from build123d import *

# Parameters (mm, degrees)
SKETCH1_R           = 10
BOSS_EXTRUDE1_DEPTH = 10


with BuildPart() as part:
    # Sketch1 → Boss-Extrude1 (new, symmetric)
    with BuildSketch(Plane.XY):
        with BuildLine():
            Line((-24.140215409, 6.5), (-11.587303396, 53.12))
            ThreePointArc((-11.587303396, 53.12), (0, 62), (11.587303396, 53.12))
            Line((11.587303396, 53.12), (24.140215409, 6.5))
            ThreePointArc((24.140215409, 6.5), (24.936514863, 1.780512988), (24.81883517, -3.004233816))
            ThreePointArc((24.81883517, -3.004233816), (30.762049538, -19.776348187), (47.717387131, -25.174694658))
            ThreePointArc((47.717387131, -25.174694658), (61.713032142, -49.370425713), (35.03522611, -41.027395935))
            ThreePointArc((35.03522611, -41.027395935), (26.046643252, -25.670606045), (8.378996809, -23.554031767))
            ThreePointArc((8.378996809, -23.554031767), (0, -25), (-8.378996809, -23.554031767))
            ThreePointArc((-8.378996809, -23.554031767), (-26.046643252, -25.670606045), (-35.03522611, -41.027395935))
            ThreePointArc((-35.03522611, -41.027395935), (-61.713032142, -49.370425713), (-47.717387131, -25.174694658))
            ThreePointArc((-47.717387131, -25.174694658), (-30.762049538, -19.776348187), (-24.81883517, -3.004233816))
            ThreePointArc((-24.81883517, -3.004233816), (-24.936514863, 1.780512988), (-24.140215409, 6.5))
        make_face()
        with Locations((-50, -40)):
            Circle(SKETCH1_R, mode=Mode.SUBTRACT)
        with Locations(Location((50, -40, 0), (0, 0, 180))):
            Circle(SKETCH1_R, mode=Mode.SUBTRACT)
        with BuildLine():
            Line((-19.078784028, 6), (-4.769696007, 51.5))
            ThreePointArc((-4.769696007, 51.5), (0, 55), (4.769696007, 51.5))
            Line((4.769696007, 51.5), (19.078784028, 6))
            ThreePointArc((19.078784028, 6), (0, -20), (-19.078784028, 6))
        make_face(mode=Mode.SUBTRACT)
    extrude(amount=BOSS_EXTRUDE1_DEPTH, both=True)


solid = part.part
CAD build for the part. Positions are in the model's coordinates, mm. A direction names the side the tool comes from. Coordinates: 2 decimals unless noted, no trailing zeros. Order: outer loops, then holes, each group sorted by start corner. A loop starts at its lowest first (then second) coordinate and runs counter-clockwise, first axis right, second up.
Item 1: Drill centre lines: L1, parallel to Y at x = 50, z = 0; L2, parallel to X at y = 41.5, z = 7.75; L3, parallel to X at y = -4, z = 7.5. Where is each one in solid material? Low to high.
Check sheet entries:
L1: y = -55 to -50, -30 to -25
L2: x = -14.72 to -7.91, 7.91 to 14.72
L3: x = -24.72 to -19.6, 19.6 to 24.72
Item 2: Band-saw the part on D-D on x = 22.5. List the corners of the cut face in (y, z).
Check sheet entries:
outline: (-23.82, -10) - (12.59, -10) - (12.59, 10) - (-23.82, 10) - close
Item 3: Band-saw the part on C-C on z = 3.5. List the corners of the cut face in (x, y).
Check sheet entries:
outline: (-47.72, -25.17) arc R15 ccw (long way) to (-35.04, -41.03) arc R20 cw to (-8.38, -23.55) arc R25 ccw to (8.38, -23.55) arc R20 cw to (35.04, -41.03) arc R15 ccw (long way) to (47.72, -25.17) arc R20 cw to (24.82, -3) arc R25 ccw to (24.14, 6.5) - (11.59, 53.12) arc R12 ccw to (-11.59, 53.12) - (-24.14, 6.5) arc R25 ccw to (-24.82, -3) arc R20 cw to start; hole circle Ø20 at (-50, -40); hole (-19.08, 6) arc R20 ccw (long way) to (19.08, 6) - (4.77, 51.5) arc R5 ccw to (-4.77, 51.5) - close; hole circle Ø20 at (50, -40)
Item 4: Two-plate mould, pull along X, no slides. Class faces 3 (the face through (52.17, -30.24, -0.14)), 4 (the face through (-17.952, 29.484, 0.14)), 5 (the face through (24.93, 1.85, 0.14)): +X half, -X half, draft (parallel to the pull), parting line (faces both ways), or undercut.
Check sheet entries:
face 3: undercut
face 4: -X half
face 5: +X half
Item 5: Band-saw the part on A-A on x = 0. List the corners of the cut face in (y, z).
Check sheet entries:
outline: (-25, -10) - (-20, -10) - (-20, 10) - (-25, 10) - close; (55, -10) - (62, -10) - (62, 10) - (55, 10) - close
Item 6: 3-axis set-ups, long thin cutter, end or side, ignore diameter. For faces 1 (the face through (-12.024, 28.432, 0.14)), 2 (the face through (0, 62, 0)): which of +Z, -Z, +X, -X, +Y, -Y reach the whole face in a straight line?
Check sheet entries:
face 1: +Z, -Z
face 2: +Z, -Z, +Y
Item 7: Band-saw the part on B-B on y = -7. List the corners of the cut face in (x, z) (3 decimals), plus the area to 3 significant figures.
Check sheet entries:
outline: (-24.737, -10) - (-18.735, -10) - (-18.735, 10) - (-24.737, 10) - close; (18.735, -10) - (24.737, -10) - (24.737, 10) - (18.735, 10) - close
area: 240 mm2
Item 8: Pin check, flat tips, straight feed: pin 1 Ø10 at (x, z) = (16, -6) entering from -Y; pin 2 Ø18 at (x, y) = (50, -40) entering from +Z; pin 3 Ø1.5 at (y, z) = (12.5, -2) entering from +X; pin 4 Ø10 at (y, z) = (-13.5, 4.5) entering from -X. Stop position of each tip, or through.
Check sheet entries:
pin 1: stops at y = -23.29
pin 2: passes through
pin 3: stops at x = 22.73
pin 4: stops at x = -29.55
